Can you work these out from the model? Positions are in its coordinate system, mm. Coordinates: 2 decimals unless noted, no trailing zeros. Order: outer loops, then holes, each group sorted by start corner. A loop starts at its lowest first (then second) coordinate and runs counter-clockwise, first axis right, second up. Notation, with made-up numbers: (67.5, 84) -> (77.5, 84) arc R24 ccw to (77.5, 109) -> close; hole circle Ø2 at (-9, 84.5). An arc over 180 degrees is marked (long way). Use a Markdown table: item, result. Add a question column.
1. For pin 1 Ø6 at (x, z) = (-549, -25.5) entering from -Y; pin 2 Ø1 at (x, y) = (-471, -71) entering from +Z, each with a flat end and sliding along its axis, tell me the tip position at first contact or that it passes through.
2. Suppose I cut it at D-D, the plane z = 28. List the corners of the cut face in (x, y) for me, then the cut area to 3 significant figures.
3. If I drill on line 1 along Z through (x, y) = (-500, -69.7); line 2 along X through (y, z) = (-69.85, -28.5); line 3 along X through (y, z) = (-70.15, -29.5), over which ranges is the centre line in solid material (lowest first)? Write a range as from..to.
4. Suppose I cut it at A-A, the plane z = -56. List the corners of the cut face in (x, y) for me.
5. Suppose I cut it at C-C, the plane y = -70.2. List the corners of the cut face in (x, z) for me.
6. Suppose I cut it at B-B, the plane x = -500. List the corners of the cut face in (y, z) for me, then the cut area to 3 significant figures.
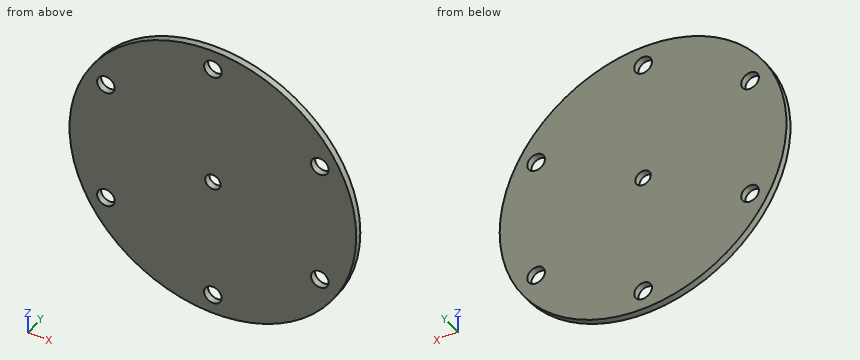
```python
from build123d import *

# Parameters (mm, degrees)
SKETCH005_R     = 65
PAD004_DEPTH    = 3
SKETCH006_R     = 4
POCKET_DEPTH    = 3.001
SKETCH011_R     = 3.5
POCKET002_DEPTH = 3.001


with BuildPart() as part:
    # Sketch005 → Pad004 (new body)
    with BuildSketch(Plane(origin=(500, 72.072, 0), x_dir=(1, 0, 0), z_dir=(0, -1, 0))):
        Circle(SKETCH005_R)
    extrude(amount=PAD004_DEPTH)

    # Sketch006 → Pocket (cut, through all)
    with BuildSketch(Plane(origin=(500, 69.072, 0), x_dir=(1, 0, 0), z_dir=(0, -1, 0))):
        with Locations((48.497423, 28)):
            Circle(SKETCH006_R)
        with Locations((48.497423, -28)):
            Circle(SKETCH006_R)
        with Locations((0, -56)):
            Circle(SKETCH006_R)
        with Locations((-48.497423, -28)):
            Circle(SKETCH006_R)
        with Locations((-48.497423, 28)):
            Circle(SKETCH006_R)
        with Locations((0, 56)):
            Circle(SKETCH006_R)
    extrude(amount=-POCKET_DEPTH, mode=Mode.SUBTRACT)


with BuildPart() as part_1:
    # Clone008 placement: moved
    add(part.part.moved(Location((-1000, -141.144, 0))))

    # Sketch011 → Pocket002 (cut, through all)
    with BuildSketch(Plane(origin=(-500, -72.072, 0), x_dir=(1, 0, 0), z_dir=(0, -1, 0))):
        Circle(SKETCH011_R)
    extrude(amount=-POCKET002_DEPTH, mode=Mode.SUBTRACT)


solid = part_1.part
```
Worked out:
| question | item | result |
|---|---|---|
| 1 | pin 1 | stops at y = -72.07 |
| 1 | pin 2 | stops at z = 58.42 |
| 2 | outline | (-558.66, -72.07) -> (-552.5, -72.07) -> (-552.5, -69.07) -> (-558.66, -69.07) -> close; (-544.5, -72.07) -> (-455.5, -72.07) -> (-455.5, -69.07) -> (-544.5, -69.07) -> close; (-447.5, -72.07) -> (-441.34, -72.07) -> (-441.34, -69.07) -> (-447.5, -69.07) -> close |
| 2 | area | 304 mm² |
| 3 | line 1 | z = -65..-60, -52..-3.5, 3.5..52, 60..65 |
| 3 | line 2 | x = -558.42..-552.47, -544.53..-455.47, -447.53..-441.58 |
| 3 | line 3 | x = -557.92..-552.21, -544.79..-455.21, -447.79..-442.08 |
| 4 | outline | (-533, -72.07) -> (-504, -72.07) -> (-504, -69.07) -> (-533, -69.07) -> close; (-496, -72.07) -> (-467, -72.07) -> (-467, -69.07) -> (-496, -69.07) -> close |
| 5 | outline | circle Ø130 at (-500, 0); hole circle Ø8 at (-548.5, -28); hole circle Ø8 at (-548.5, 28); hole circle Ø8 at (-500, -56); hole circle Ø8 at (-500, 56); hole circle Ø7 at (-500, 0); hole circle Ø8 at (-451.5, -28); hole circle Ø8 at (-451.5, 28) |
| 6 | outline | (-72.07, -65) -> (-69.07, -65) -> (-69.07, -60) -> (-72.07, -60) -> close; (-72.07, -52) -> (-69.07, -52) -> (-69.07, -3.5) -> (-72.07, -3.5) -> close; (-72.07, 3.5) -> (-69.07, 3.5) -> (-69.07, 52) -> (-72.07, 52) -> close; (-72.07, 60) -> (-69.07, 60) -> (-69.07, 65) -> (-72.07, 65) -> close |
| 6 | area | 321 mm² |
